from build123d import *

# Parameters (mm, degrees)
F1_DEPTH  = 6
F3_DEPTH  = 20
F5_DEPTH  = 40
F7_DEPTH  = 60
F9_DEPTH  = 2
F12_R     = 3.25
F12_R_2   = 2.25
F13_DEPTH = 8.001
F14_SIZE  = 3


with BuildPart() as f1:
    # F0 (on Top) → F1 (new body)
    with BuildSketch(Plane.XY):
        Polygon((0, 66), (0, 0), (66, 0), (66, 26), (26, 26), (26, 66), align=None)
    extrude(amount=F1_DEPTH)

    # F2 (on face) → F3 (join)
    with BuildSketch(Plane.XY.offset(6)):
        Polygon((6, 66), (0, 66), (0, 0), (66, 0), (66, 6), (6, 6), align=None)
    extrude(amount=F3_DEPTH)

    # F4 (on face) → F5 (join)
    with BuildSketch(Plane.XY.offset(26)):
        Polygon((6, 6), (6, 26), (0, 26), (0, 0), (26, 0), (26, 6), align=None)
    extrude(amount=F5_DEPTH)

    # F6 (on face) → F7 (join)
    with BuildSketch(Plane.XY.offset(6)):
        Polygon((13.29, 6), (16, 6), (18.71, 6), (18.71, 8), (13.29, 8), align=None)
        Polygon((6, 18.71), (6, 16), (6, 13.29), (8, 13.29), (8, 18.71), align=None)
    extrude(amount=F7_DEPTH)

    # F8 (on face) → F9 (join)
    with BuildSketch(Plane.XY.offset(6)):
        Polygon((66, 13.29), (66, 16), (66, 18.71), (26, 18.71), (26, 13.29), align=None)
        Polygon((18.71, 66), (16, 66), (13.29, 66), (13.29, 26), (18.71, 26), align=None)
    extrude(amount=F9_DEPTH)

    # F12 (on face) → F13 (cut, through all)
    with BuildSketch(Plane(origin=(0, 0, 0), x_dir=(1, 0, 0), z_dir=(0, 0, -1))):
        with Locations((16, -16)):
            Circle(F12_R)
        with Locations((46, -16)):
            Circle(F12_R_2)
        with Locations((16, -46)):
            Circle(F12_R_2)
    extrude(amount=-F13_DEPTH, mode=Mode.SUBTRACT)

    # F14
    f14_edges = [f1.edges().sort_by_distance(p)[0] for p in [
        (0, 0, 33),
        (0, 26, 46),
        (0, 46, 26),
        (26, 0, 46),
        (46, 0, 26),
        (0, 13, 66),
        (13, 0, 66),
        (0, 66, 13),
        (66, 0, 13),
    ]]
    chamfer(f14_edges, length=F14_SIZE)


solid = f1.part
Input: part model. Units: mm. Frame: model coordinates. A direction names the side the tool comes from. Give positions to 0.01 mm unless a question says otherwise; leave off trailing zeros. Order: outer loops, then holes, each group sorted by start corner. A loop starts at its lowest first (then second) coordinate and runs counter-clockwise, first axis right, second up. Notation, with made-up numbers: M -9,24.5 L 42,24.5 A23 ccw 42,43.5 Z; hole C 7,34 d5. An arc over 180 degrees is marked long. Answer as a JSON object with one key per item and string values.
1. Pull-direction query (X, two-part tool) for faces 5 (the flat face through (46, 5, 26)), 6 (the flat face through (0, 20, 24)), 7 (the cylindrical face through (43.752, 15.901, 3.944)); classes: +X half, -X half, draft (parallel to the pull), parting line (faces both ways), or undercut.
Result sheet:
{"face 5": "draft", "face 6": "-X half", "face 7": "undercut"}
2. Cut plane A-A, the plane x = 16. Output: boundary loops of the cut face in (y, z), and give its area (4 significant figures).
Result sheet:
{"outline": "M 0,0 L 12.75,0 L 12.75,6 L 8,6 L 8,66 L 3,66 L 0,63 Z; M 19.25,0 L 43.75,0 L 43.75,8 L 26,8 L 26,6 L 19.25,6 Z; M 48.25,0 L 66,0 L 66,8 L 48.25,8 Z", "area": "876.5 mm²"}
3. Ray query, line 1 (Y direction, x = 16, z = 1); line 2 (Y direction, x = 7, z = 48). Return the intervals inside material, ascending. Write a range as [from, to].
Result sheet:
{"line 1": "[0, 12.75], [19.25, 43.75], [48.25, 66]", "line 2": "[0, 6], [13.29, 18.71]"}
4. Reachability of faces 1 (the flat face through (13.29, 46, 7)), 2 (the flat face through (46, 26, 3)), 3 (the flat face through (18.71, 7, 36)), 4 (the flat face through (1, 24, 44)) from +Z, -Z, +X, -X, +Y, -Y: full face, straight path, thin tool, end or side. Return the list, or none.
Result sheet:
{"face 1": "+Z, +Y", "face 2": "+Z, -Z, +X, +Y", "face 3": "+Z, +X, +Y", "face 4": "+Z, -X, +Y"}
5. First-contact query: P1, Ø2.5, axis at x = 37.5, y = 5, coming from the +Z side; P2, Ø0.6, axis at y = 54.5, z = 6.5, coming from the +X side; P3, Ø1.6, axis at y = 6.5, z = 50, coming from the +X side. Flat tips, straight axial feed; report the tip coordinate or a pass-through.
Result sheet:
{"P1": "z = 26", "P2": "x = 18.71", "P3": "x = 26"}
6. Cut plane B-B, the plane y = 46. Output: boundary loops of the cut face in (x, z), and give its area (3 significant figures).
Result sheet:
{"outline": "M 0,0 L 13.75,0 L 13.75,8 L 13.29,8 L 13.29,6 L 6,6 L 6,26 L 3,26 L 0,23 Z; M 18.25,0 L 26,0 L 26,6 L 18.71,6 L 18.71,8 L 18.25,8 Z", "area": "246 mm²"}
